For this review, take the finished solid that the model builds, in its own axes (mm). Face numbers are marked on the shaded views. A direction names the side the tool comes from. Round coordinates to 2 decimals unless told otherwise and drop trailing zeros. Loops run counter-clockwise (first coordinate to the right, second up) from the corner with the lowest first, then second, coordinate; pieces in that order, holes last.
1) Wall thickness on L1, parallel to X at y = 8, z = 0; L2, parallel to X at y = 8.5, z = -20; L3, parallel to Z at x = 15.5, y = 8: over which ranges is each line inside the solid? List them lowest first.
2) Take a section at D-D (x = -21). State the section outline as (y, z) points.
3) Mouldability with a two-part tool opening along Z and no side actions: class the marked faces 3, 4 and 5 as pulls with the +Z half, pulls with the -Z half, needs draft (parallel to the pull), parting line crosses it, or undercut.
4) Take a section at A-A (y = 1). State the section outline as (x, z) points, then the cut area to 3 significant figures.
5) Insertion check: pin 1 (2 mm diameter, centred on x = 19.5, y = 4.5, fed in from +Z); pin 2 (6 mm diameter, centred on x = 2, z = -0.5, fed in from +Y). Each pin has a flat end and moves straight along its axis. Give the tip position at first contact, or say it passes through.
6) Take a section at B-B (x = 0). State the section outline as (y, z) points, then the cut area to 3 significant figures.
7) Take a section at C-C (z = -20). State the section outline as (x, y) points.
8) Tool access review of the marked faces 1 and 2: name each direction out of +Z, -Z, +X, -X, +Y, -Y from which nothing blocks a thin tool from reaching the whole face with its end or side.
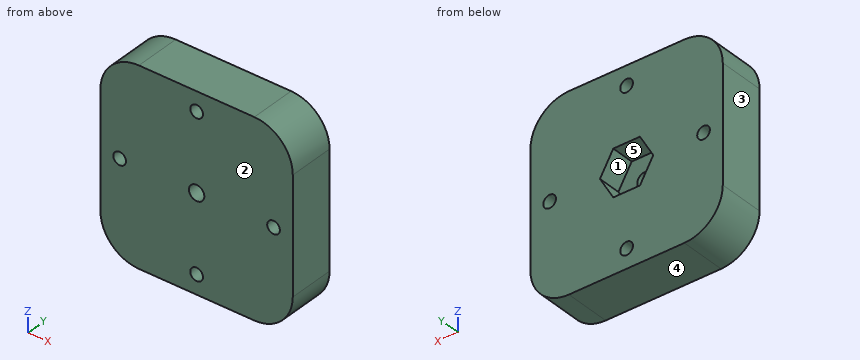
```python
from build123d import *

# Parameters (mm, degrees)
SKETCH1_W           = 50
SKETCH1_H           = 50
BOSS_EXTRUDE1_DEPTH = 12
CUT_EXTRUDE1_DEPTH  = 6
SKETCH4_R           = 1.65
CUT_EXTRUDE2_DEPTH  = 25
FILLET1_R           = 10
SKETCH5_R           = 2
CUT_EXTRUDE4_DEPTH  = 10


with BuildPart() as part:
    # Sketch1 → Boss-Extrude1 (new body)
    with BuildSketch(Plane(origin=(0, 0, 0), x_dir=(1, 0, 0), z_dir=(0, 1, 0))):
        Rectangle(SKETCH1_W, SKETCH1_H)
    extrude(amount=BOSS_EXTRUDE1_DEPTH)

    # Sketch2 → Cut-Extrude1 (cut)
    with BuildSketch(Plane(origin=(0, 12, 0), x_dir=(1, 0, 0), z_dir=(0, 1, 0))):
        Polygon((6.92820323, 0), (3.464101615, 6), (-3.464101615, 6), (-6.92820323, 0), (-3.464101615, -6), (3.464101615, -6), align=None)
    extrude(amount=-CUT_EXTRUDE1_DEPTH, mode=Mode.SUBTRACT)

    # Sketch4 → Cut-Extrude2 (cut)
    with BuildSketch(Plane(origin=(0, 12, 0), x_dir=(1, 0, 0), z_dir=(0, 1, 0))):
        with Locations(Location((0, 20, 0), (0, 0, 270))):
            Circle(SKETCH4_R)
        with Locations(Location((20, 0, 0), (0, 0, 270))):
            Circle(SKETCH4_R)
        with Locations(Location((-20, 0, 0), (0, 0, 270))):
            Circle(SKETCH4_R)
        with Locations(Location((0, -20, 0), (0, 0, 270))):
            Circle(SKETCH4_R)
    extrude(amount=-CUT_EXTRUDE2_DEPTH, mode=Mode.SUBTRACT)

    # Fillet1
    fillet1_edges = [part.edges().sort_by_distance(p)[0] for p in [
        (25, 6, 25),
        (-25, 6, 25),
        (-25, 6, -25),
        (25, 6, -25),
    ]]
    fillet(fillet1_edges, radius=FILLET1_R)

    # Sketch5 → Cut-Extrude4 (cut)
    with BuildSketch(Plane(origin=(0, 0, 0), x_dir=(1, 0, 0), z_dir=(0, 1, 0))):
        with Locations(Location((0, 0, 0), (0, 0, 270))):
            Circle(SKETCH5_R)
    extrude(amount=CUT_EXTRUDE4_DEPTH, mode=Mode.SUBTRACT)


solid = part.part
```
Response:
1. L1: x = -25 to -21.65, -18.35 to -6.93, 6.93 to 18.35, 21.65 to 25
1. L2: x = -23.66 to -1.65, 1.65 to 23.66
1. L3: z = -24.99 to 24.99
2. outline: (0, -23) - (12, -23) - (12, -1.31) - (0, -1.31) - close; (0, 1.31) - (12, 1.31) - (12, 23) - (0, 23) - close
3. face 3: needs draft
3. face 4: pulls with the -Z half
3. face 5: undercut
4. outline: (-25, -15) arc R10 ccw to (-15, -25) - (15, -25) arc R10 ccw to (25, -15) - (25, 15) arc R10 ccw to (15, 25) - (-15, 25) arc R10 ccw to (-25, 15) - close; hole circle Ø3.3 at (-20, 0); hole circle Ø4 at (0, 0); hole circle Ø3.3 at (0, -20); hole circle Ø3.3 at (0, 20); hole circle Ø3.3 at (20, 0)
4. area: 2,370 mm2
5. pin 1: stops at z = 24.37
5. pin 2: stops at y = 6
6. outline: (0, -25) - (12, -25) - (12, -21.65) - (0, -21.65) - close; (0, -18.35) - (12, -18.35) - (12, -6) - (6, -6) - (6, -2) - (0, -2) - close; (0, 2) - (6, 2) - (6, 6) - (12, 6) - (12, 18.35) - (0, 18.35) - close; (0, 21.65) - (12, 21.65) - (12, 25) - (0, 25) - close
6. area: 425 mm2
7. outline: (-23.66, 0) - (-1.65, 0) - (-1.65, 12) - (-23.66, 12) - close; (1.65, 0) - (23.66, 0) - (23.66, 12) - (1.65, 12) - close
8. face 1: +Y
8. face 2: +Z, -Z, +X, -X, -Y
